Can you work these out from the model? Positions are in its coordinate system, mm. Round coordinates to 2 decimals unless told otherwise and drop trailing zeros. Loops run counter-clockwise (first coordinate to the right, second up) from the corner with the lowest first, then second, coordinate; pieces in that order, holes last. Notation, with made-up numbers: (-4.75, -1.75) -> (11.25, -1.75) arc R25 cw to (11.25, 14.25) -> close; hole circle Ø7 at (32.25, 9.25). An arc over 180 degrees is marked (long way). Write each question's results on one line, items separated by ' | '.
Autodesk Inventor part; units mm, degrees
ref_plane "YZ Plane" through (0, 0, 0) normal (1, 0, 0) x (0, 1, 0)
ref_plane "XZ Plane" through (0, 0, 0) normal (0, 1, 0) x (-1, 0, 0)
ref_plane "XY Plane" through (0, 0, 0) normal (0, 0, 1) x (1, 0, 0)
sketch "Szkic1" plane through (0, 0, 0) normal (0, 0, 1) x (1, 0, 0)
  line L0 (-9.375, -9.875) -> (9.375, -9.875)
  line L1 (12.375, -6.875) -> (12.375, 6.875)
  line L2 (9.375, 9.875) -> (-9.375, 9.875)
  line L3 (-12.375, 6.875) -> (-12.375, -6.875)
  arc A0 (-9.375, 9.875) -> (-12.375, 6.875) centre (-9.375, 6.875) ccw
  arc A1 (12.375, 6.875) -> (9.375, 9.875) centre (9.375, 6.875) ccw
  arc A2 (9.375, -9.875) -> (12.375, -6.875) centre (9.375, -6.875) ccw
  arc A3 (-12.375, -6.875) -> (-9.375, -9.875) centre (-9.375, -6.875) ccw
  point P0 (0, 0)
  point P1 (12.375, 9.875)
  point P2 (12.375, -9.875)
  point P3 (-12.375, 9.875)
  dimension "d0" = 24.75
  dimension "d1" = 19.75
  dimension "d2" = 3
extrude "Wyciągnięcie proste1" add sketch "Szkic1" along normal blind 1.5
properties part number "PODUSZKA PODSTAWY" material "Kauczuk, silikon"
1. If we section it at A-A (z = 0.85): List the corners of the cut face in (x, y) for me (3 decimals).
Final values:
outline: (-12.375, -6.875) arc R3 ccw to (-9.375, -9.875) -> (9.375, -9.875) arc R3 ccw to (12.375, -6.875) -> (12.375, 6.875) arc R3 ccw to (9.375, 9.875) -> (-9.375, 9.875) arc R3 ccw to (-12.375, 6.875) -> close
2. Please list where these lines run through material, in increasing order: line 1 (X direction, y = -7, z = 1.4); line 2 (X direction, y = 9.25, z = 0.6); line 3 (Y direction, x = -10, z = 1.4). Write a range as from..to.
Final values:
line 1: -12.37..12.37 | line 2: -11.21..11.21 | line 3: -9.81..9.81
3. If we section it at B-B (x = -10.5): List the corners of the cut face in (y, z) for me, then the cut area to 3 significant figures.
Final values:
outline: (-9.66, 0) -> (9.66, 0) -> (9.66, 1.5) -> (-9.66, 1.5) -> close | area: 29.0 mm2
